Work out the finished part from the listing and answer in its coordinate system (mm). Coordinates: 2 decimals unless noted, no trailing zeros. Order: outer loops, then holes, each group sorted by start corner. A loop starts at its lowest first (then second) coordinate and runs counter-clockwise, first axis right, second up. Notation, with made-up numbers: (81, 77.5) -> (139, 77.5) arc R21 ccw to (139, 116.5) -> close; hole circle Ø11 at (83, 71). An arc over 180 degrees is marked (long way). Answer as CSV lines item,"result". Start each with the question number.
Item 1: Each of these flat-tipped pins is pushed along its axis until it touches: pin 1 Ø3 at (x, y) = (0, 0) entering from -Z; pin 2 Ø1 at (x, y) = (0, 0) entering from +Z. Where does it stop, or does it pass through?
Item 2: Section D-D (y = 4.75) is taken. Write down the section's boundary in (x, z).
Item 3: Straight lines are drawn through the part: L1, parallel to Y at x = 0, z = 56.5; L2, parallel to Y at x = 0, z = 4.5 (3 decimals); L3, parallel to X at y = 0, z = 4.75 (3 decimals). For each, find the intervals that lie inside material, in ascending order.
Item 4: Section B-B (x = 0) is taken. Write down the section's boundary in (y, z) (3 decimals).
Item 5: Section C-C (z = 26.5) is taken. Write down the section's boundary in (x, y), then the cut area to 3 significant figures.
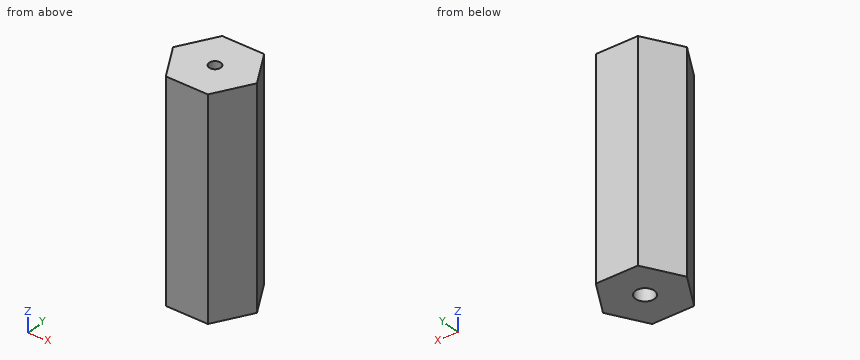
Autodesk Fusion 360 part; units mm, degrees
sketch "Sketch1" plane through (0, 0, 0) normal (0, 0, 1) x (1, 0, 0)
  line L0 (-5.7735, 10) -> (-11.547, 0)
  line L1 (-11.547, 0) -> (-5.7735, -10)
  line L2 (-5.7735, -10) -> (5.7735, -10)
  line L3 (5.7735, -10) -> (11.547, 0)
  line L4 (11.547, 0) -> (5.7735, 10)
  line L5 (5.7735, 10) -> (-5.7735, 10)
  dimension "d1" = 10
extrude "Extrude1" add sketch "Sketch1" along normal blind 60
sketch "Sketch2" plane through (0, 0, 60) normal (0, 0, 1) x (-1, 0, 0)
  line L0 (-5.7735, -10) -> (5.7735, -10)
  line L1 (5.7735, -10) -> (11.547, 0)
  line L2 (11.547, 0) -> (5.7735, 10)
  line L3 (5.7735, 10) -> (-5.7735, 10)
  line L4 (-5.7735, 10) -> (-11.547, 0)
  line L5 (-11.547, 0) -> (-5.7735, -10)
  circle A0 centre (0, 0) radius 1.6
  dimension "d4" = 3.2
extrude "Extrude3" cut sketch "Sketch2" against normal blind 10 contours A0
sketch "Sketch4" plane through (0, 0, 0) normal (0, 0, -1) x (1, 0, 0)
  line L0 (-5.7735, -10) -> (5.7735, -10)
  line L1 (5.7735, -10) -> (11.547, 0)
  line L2 (11.547, 0) -> (5.7735, 10)
  line L3 (5.7735, 10) -> (-5.7735, 10)
  line L4 (-5.7735, 10) -> (-11.547, 0)
  line L5 (-11.547, 0) -> (-5.7735, -10)
  circle A0 centre (0, 0) radius 2.625
  dimension "d9" = 5.25
extrude "Extrude4" cut sketch "Sketch4" against normal blind 10 contours A0
Checked values:
1,pin 1,"stops at z = 10"
1,pin 2,"stops at z = 50"
2,outline,"(-8.8, 0) -> (8.8, 0) -> (8.8, 60) -> (-8.8, 60) -> close"
3,L1,"y = -10 to -1.6, 1.6 to 10"
3,L2,"y = -10 to -2.625, 2.625 to 10"
3,L3,"x = -11.547 to -2.625, 2.625 to 11.547"
4,outline,"(-10, 0) -> (-2.625, 0) -> (-2.625, 10) -> (2.625, 10) -> (2.625, 0) -> (10, 0) -> (10, 60) -> (1.6, 60) -> (1.6, 50) -> (-1.6, 50) -> (-1.6, 60) -> (-10, 60) -> close"
5,outline,"(-11.55, 0) -> (-5.77, -10) -> (5.77, -10) -> (11.55, 0) -> (5.77, 10) -> (-5.77, 10) -> close"
5,area,"346 mm^2"
